Part model, mm, in its own coordinate system. Face numbers are marked on the shaded views. A direction names the side the tool comes from. Give positions to 0.01 mm unless a question says otherwise; leave off trailing zeros. Order: outer loops, then holes, each group sorted by start corner. A loop starts at its lowest first (then second) coordinate and runs counter-clockwise, first axis right, second up. Notation, with made-up numbers: (86.5, 79.5) - (126.5, 79.5) arc R31 cw to (126.5, 103.5) - close; hole circle Ø6 at (-22.5, 73). An arc over 180 degrees is marked (long way). One line per item, written item: value.
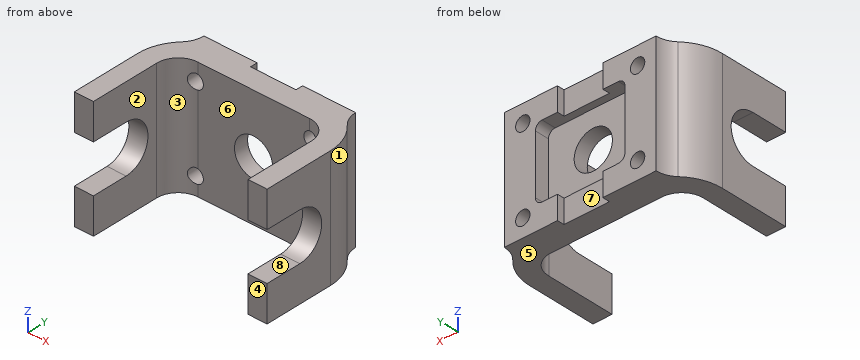
```python
from build123d import *

# Parameters (mm, degrees)
BOSS_EXTRUDE1_DEPTH = 31.75
CUT_EXTRUDE1_DEPTH  = 103.362
CUT_EXTRUDE2_DEPTH  = 7.62
SKETCH5_W           = 24.13
SKETCH5_H           = 3.81
CUT_EXTRUDE3_DEPTH  = 64.5
CUT_EXTRUDE4_REACH  = 57.88
SKETCH6_R           = 10.16
CUT_EXTRUDE5_REACH  = 65.5
SKETCH7_R           = 3.81


with BuildPart() as part:
    # Sketch2 → Boss-Extrude1 (new body, symmetric)
    with BuildSketch(Plane.XY):
        with BuildLine():
            Line((-29.591, 0), (29.591, 0))
            ThreePointArc((29.591, 0), (37.673230509, -3.347769491), (41.021, -11.43))
            Line((41.021, -11.43), (41.021, -48.26))
            Line((41.021, -48.26), (51.181, -48.26))
            Line((51.181, -48.26), (51.181, -11.43))
            ThreePointArc((51.181, -11.43), (49.29585059, -1.827302371), (43.920228208, 6.35))
            ThreePointArc((43.920228208, 6.35), (41.232417018, 10.438651186), (40.289842313, 15.24))
            Line((40.289842313, 15.24), (-40.289842313, 15.24))
            ThreePointArc((-40.289842313, 15.24), (-41.232417018, 10.438651186), (-43.920228208, 6.35))
            ThreePointArc((-43.920228208, 6.35), (-49.29585059, -1.827302371), (-51.181, -11.43))
            Line((-51.181, -11.43), (-51.181, -48.26))
            Line((-51.181, -48.26), (-41.021, -48.26))
            Line((-41.021, -48.26), (-41.021, -11.43))
            ThreePointArc((-41.021, -11.43), (-37.673230509, -3.347769491), (-29.591, 0))
        make_face()
    extrude(amount=BOSS_EXTRUDE1_DEPTH, both=True)

    # Sketch3 → Cut-Extrude1 (cut, through all)
    with BuildSketch(Plane(origin=(51.181, 0, 0), x_dir=(0, 0, -1), z_dir=(1, 0, 0))):
        with BuildLine():
            Line((-12.7, -48.26), (12.7, -48.26))
            Line((12.7, -48.26), (12.7, -29.21))
            ThreePointArc((12.7, -29.21), (0, -16.51), (-12.7, -29.21))
            Line((-12.7, -29.21), (-12.7, -48.26))
        make_face()
    extrude(amount=-CUT_EXTRUDE1_DEPTH, mode=Mode.SUBTRACT)

    # Sketch4 → Cut-Extrude2 (cut)
    with BuildSketch(Plane(origin=(0, 15.24, 0), x_dir=(1, 0, 0), z_dir=(0, 1, 0))):
        with BuildLine():
            Line((-20.223842313, 19.304), (20.223842313, 19.304))
            ThreePointArc((20.223842313, 19.304), (22.738314027, 18.262471714), (23.779842313, 15.748))
            Line((23.779842313, 15.748), (23.779842313, -15.748))
            ThreePointArc((23.779842313, -15.748), (22.738314027, -18.262471714), (20.223842313, -19.304))
            Line((20.223842313, -19.304), (-20.223842313, -19.304))
            ThreePointArc((-20.223842313, -19.304), (-22.738314027, -18.262471714), (-23.779842313, -15.748))
            Line((-23.779842313, -15.748), (-23.779842313, 15.748))
            ThreePointArc((-23.779842313, 15.748), (-22.738314027, 18.262471714), (-20.223842313, 19.304))
        make_face()
    extrude(amount=-CUT_EXTRUDE2_DEPTH, mode=Mode.SUBTRACT)

    # Sketch5 → Cut-Extrude3 (cut, through all)
    with BuildSketch(Plane.XY.offset(31.75)):
        with Locations((0, 13.335)):
            Rectangle(SKETCH5_W, SKETCH5_H)
    extrude(amount=-CUT_EXTRUDE3_DEPTH, mode=Mode.SUBTRACT)

    # Sketch6 → Cut-Extrude4 (cut, up to next)
    with BuildSketch(Plane(origin=(0, 7.62, 0), x_dir=(1, 0, 0), z_dir=(0, 1, 0)), mode=Mode.PRIVATE) as cut_extrude4_sk1:
        Circle(SKETCH6_R)
    cut_extrude4_tool1 = extrude(cut_extrude4_sk1.sketch, amount=-CUT_EXTRUDE4_REACH, mode=Mode.PRIVATE) & part.part
    add(cut_extrude4_tool1.solids().sort_by_distance((0, 7.62, 0))[0], mode=Mode.SUBTRACT)

    # Sketch7 → Cut-Extrude5 (cut, up to next)
    with BuildSketch(Plane(origin=(0, 15.24, 0), x_dir=(1, 0, 0), z_dir=(0, 1, 0)), mode=Mode.PRIVATE) as cut_extrude5_sk1:
        with Locations((-30.48, 22.225)):
            Circle(SKETCH7_R)
    cut_extrude5_tool1 = extrude(cut_extrude5_sk1.sketch, amount=-CUT_EXTRUDE5_REACH, mode=Mode.PRIVATE) & part.part
    add(cut_extrude5_tool1.solids().sort_by_distance((-30.48, 15.24, -22.225))[0], mode=Mode.SUBTRACT)
    # Sketch7 → Cut-Extrude5 (cut, up to next)
    with BuildSketch(Plane(origin=(0, 15.24, 0), x_dir=(1, 0, 0), z_dir=(0, 1, 0)), mode=Mode.PRIVATE) as cut_extrude5_sk2:
        with Locations((30.48, 22.225)):
            Circle(SKETCH7_R)
    cut_extrude5_tool2 = extrude(cut_extrude5_sk2.sketch, amount=-CUT_EXTRUDE5_REACH, mode=Mode.PRIVATE) & part.part
    add(cut_extrude5_tool2.solids().sort_by_distance((30.48, 15.24, -22.225))[0], mode=Mode.SUBTRACT)
    # Sketch7 → Cut-Extrude5 (cut, up to next)
    with BuildSketch(Plane(origin=(0, 15.24, 0), x_dir=(1, 0, 0), z_dir=(0, 1, 0)), mode=Mode.PRIVATE) as cut_extrude5_sk3:
        with Locations((30.48, -22.225)):
            Circle(SKETCH7_R)
    cut_extrude5_tool3 = extrude(cut_extrude5_sk3.sketch, amount=-CUT_EXTRUDE5_REACH, mode=Mode.PRIVATE) & part.part
    add(cut_extrude5_tool3.solids().sort_by_distance((30.48, 15.24, 22.225))[0], mode=Mode.SUBTRACT)
    # Sketch7 → Cut-Extrude5 (cut, up to next)
    with BuildSketch(Plane(origin=(0, 15.24, 0), x_dir=(1, 0, 0), z_dir=(0, 1, 0)), mode=Mode.PRIVATE) as cut_extrude5_sk4:
        with Locations((-30.48, -22.225)):
            Circle(SKETCH7_R)
    cut_extrude5_tool4 = extrude(cut_extrude5_sk4.sketch, amount=-CUT_EXTRUDE5_REACH, mode=Mode.PRIVATE) & part.part
    add(cut_extrude5_tool4.solids().sort_by_distance((-30.48, 15.24, 22.225))[0], mode=Mode.SUBTRACT)


solid = part.part
```
1) Drill centre lines: line 1 along Z through (x, y) = (-30.48, 5.25) (3 decimals); line 2 along X through (y, z) = (-12.5, -23); line 3 along X through (y, z) = (6, 21). Where is each one in solid material? Low to high. Write a range as from..to.
Outcome:
line 1: z = -31.75..-26.035, -18.415..18.415, 26.035..31.75
line 2: x = -51.18..-41.02, 41.02..51.18
line 3: x = -44.26..-34.09, -26.87..26.87, 34.09..44.26
2) Cut at C-C, the plane z = 5. Give the cut face in (x, y), then the cut area to 3 significant figures.
Outcome:
outline: (-51.18, -17.54) - (-41.02, -17.54) - (-41.02, -11.43) arc R11.43 cw to (-29.59, 0) - (-8.84, 0) - (-8.84, 7.62) - (-23.78, 7.62) - (-23.78, 15.24) - (-40.29, 15.24) arc R12.7 cw to (-43.92, 6.35) arc R25.4 ccw to (-51.18, -11.43) - close; (8.84, 0) - (29.59, 0) arc R11.43 cw to (41.02, -11.43) - (41.02, -17.54) - (51.18, -17.54) - (51.18, -11.43) arc R25.4 ccw to (43.92, 6.35) arc R12.7 cw to (40.29, 15.24) - (23.78, 15.24) - (23.78, 7.62) - (8.84, 7.62) - close
area: 1,220 mm^2
3) Pin check, flat tips, straight feed: pin 1 (4 mm diameter, centred on y = 12.5, z = -25, fed in from +X); pin 2 (1.9 mm diameter, centred on y = 14, z = -23, fed in from -X); pin 3 (11.5 mm diameter, centred on x = 0.5, z = -8.5, fed in from +Y). Stop position of each tip, or through.
Outcome:
pin 1: stops at x = 41.21
pin 2: stops at x = -40.48
pin 3: stops at y = 7.62
4) Cut at A-A, the plane x = 0. Give the cut face in (y, z).
Outcome:
outline: (0, -31.75) - (11.43, -31.75) - (11.43, -19.3) - (7.62, -19.3) - (7.62, -10.16) - (0, -10.16) - close; (0, 10.16) - (7.62, 10.16) - (7.62, 19.3) - (11.43, 19.3) - (11.43, 31.75) - (0, 31.75) - close
5) Which spindle directions (+Z, -Z, +X, -X, +Y, -Y) get a long thin tool onto all of the face, cutting with end or side? Do the marked faces 5, 6, 7 and 8. Say none if no direction does.
Outcome:
face 5: -Z, +X, -X, +Y, -Y
face 6: +Z, -Z, -Y
face 7: +Z, -Z, +Y
face 8: +X, -X, -Y
6) Cut at D-D, the plane x = -17.5. Give the cut face in (y, z).
Outcome:
outline: (0, -31.75) - (15.24, -31.75) - (15.24, -19.3) - (7.62, -19.3) - (7.62, 19.3) - (15.24, 19.3) - (15.24, 31.75) - (0, 31.75) - close
7) Mould opens along X. For the marked faces 1, 2, 3 and 4 say: released by +X, released by -X, zero draft, split by the parting line, or undercut.
Outcome:
face 1: released by +X
face 2: undercut
face 3: undercut
face 4: zero draft
8) Cut at B-B, the plane y = -37.5. Give the cut face in (x, z).
Outcome:
outline: (-51.18, -31.75) - (-41.02, -31.75) - (-41.02, -12.7) - (-51.18, -12.7) - close; (-51.18, 12.7) - (-41.02, 12.7) - (-41.02, 31.75) - (-51.18, 31.75) - close; (41.02, -31.75) - (51.18, -31.75) - (51.18, -12.7) - (41.02, -12.7) - close; (41.02, 12.7) - (51.18, 12.7) - (51.18, 31.75) - (41.02, 31.75) - close
